Read the model definition and answer for the solid it produces. Units are mm, in the model's axes. A direction names the side the tool comes from. Coordinates: 2 decimals unless noted, no trailing zeros. Loops run counter-clockwise (first coordinate to the right, second up) from the corner with the lowest first, then second, coordinate; pieces in that order, holes last. Notation, with made-up numbers: M -19,45 L 4,45 A32 cw 4,80 Z; hole C -17.5,-34.5 d8. An arc over 180 degrees is marked long. One line per item, written item: value. Start each with the question number.
```python
from build123d import *

# Parameters (mm, degrees)
EXTRUDE_1_DEPTH     = 3
FILLET_1_R          = 5
SKETCH_4_R          = 1.75
SKETCH_4_R_2        = 1.35
CUT_EXTRUDE_2_DEPTH = 10
CUT_EXTRUDE_3_DEPTH = 10
SKETCH_5_R          = 1.6
CUT_EXTRUDE_4_DEPTH = 10


with BuildPart() as part:
    # Sketch 1 → Extrude 1 (new body)
    with BuildSketch(Plane(origin=(0, 0, 0), x_dir=(1, 0, 0), z_dir=(0, 1, 0))):
        Polygon((-84.734156599, 82.359506041), (109.265843401, 82.359506041), (109.265843401, 107.359506041), (137.265843401, 107.359506041), (137.265843401, 82.359506041), (137.265843401, -67.640493959), (-112.734156599, -67.640493959), (-112.734156599, 55.552013884), (-112.734156599, 107.359506041), (-84.734156599, 107.359506041), align=None)
    extrude(amount=EXTRUDE_1_DEPTH)

    # Fillet 1
    fillet_1_edges = [part.edges().sort_by_distance(p)[0] for p in [
        (137.265843401, 1.5, 67.640493959),
        (-112.734156599, 1.5, 67.640493959),
        (-112.734156599, 1.5, -107.359506041),
        (-84.734156599, 1.5, -107.359506041),
        (-84.734156599, 1.5, -82.359506041),
        (109.265843401, 1.5, -82.359506041),
        (109.265843401, 1.5, -107.359506041),
        (137.265843401, 1.5, -107.359506041),
    ]]
    fillet(fillet_1_edges, radius=FILLET_1_R)

    # Sketch 4 → Cut-Extrude 2 (cut)
    with BuildSketch(Plane(origin=(0, 3, 0), x_dir=(1, 0, 0), z_dir=(0, 1, 0))):
        with Locations(Location((12.608682616, 49.5, 0), (0, 0, 270))):
            Circle(SKETCH_4_R)
        with Locations(Location((-18.891317384, -14.5, 0), (0, 0, 270))):
            Circle(SKETCH_4_R)
        with Locations(Location((-42.582797937, 49.995, 0), (0, 0, 270))):
            Circle(SKETCH_4_R_2)
        with Locations(Location((-78.582797937, 13.995, 0), (0, 0, 270))):
            Circle(SKETCH_4_R_2)
        with Locations(Location((-42.582797937, 13.995, 0), (0, 0, 270))):
            Circle(SKETCH_4_R_2)
        with Locations(Location((12.608682616, -14.5, 0), (0, 0, 270))):
            Circle(SKETCH_4_R)
        with Locations(Location((-18.891317384, 49.5, 0), (0, 0, 270))):
            Circle(SKETCH_4_R)
        with Locations(Location((-78.582797937, 49.995, 0), (0, 0, 270))):
            Circle(SKETCH_4_R_2)
    extrude(amount=-CUT_EXTRUDE_2_DEPTH, mode=Mode.SUBTRACT)

    # Sketch 4_3 → Cut-Extrude 3 (cut)
    with BuildSketch(Plane(origin=(0, 3, 0), x_dir=(1, 0, 0), z_dir=(0, 1, 0))):
        with BuildLine():
            Line((57.265843401, 74.859506041), (107.265843401, 74.859506041))
            ThreePointArc((107.265843401, 74.859506041), (109.765843401, 72.359506041), (107.265843401, 69.859506041))
            Line((107.265843401, 69.859506041), (57.265843401, 69.859506041))
            ThreePointArc((57.265843401, 69.859506041), (54.765843401, 72.359506041), (57.265843401, 74.859506041))
        make_face()
        with BuildLine():
            Line((57.265843401, 59.859506041), (107.265843401, 59.859506041))
            ThreePointArc((107.265843401, 59.859506041), (109.765843401, 57.359506041), (107.265843401, 54.859506041))
            Line((107.265843401, 54.859506041), (57.265843401, 54.859506041))
            ThreePointArc((57.265843401, 54.859506041), (54.765843401, 57.359506041), (57.265843401, 59.859506041))
        make_face()
        with BuildLine():
            Line((57.265843401, 44.859506041), (107.265843401, 44.859506041))
            ThreePointArc((107.265843401, 44.859506041), (109.765843401, 42.359506041), (107.265843401, 39.859506041))
            Line((107.265843401, 39.859506041), (57.265843401, 39.859506041))
            ThreePointArc((57.265843401, 39.859506041), (54.765843401, 42.359506041), (57.265843401, 44.859506041))
        make_face()
        with BuildLine():
            Line((57.265843401, 29.859506041), (107.265843401, 29.859506041))
            ThreePointArc((107.265843401, 29.859506041), (109.765843401, 27.359506041), (107.265843401, 24.859506041))
            Line((107.265843401, 24.859506041), (57.265843401, 24.859506041))
            ThreePointArc((57.265843401, 24.859506041), (54.765843401, 27.359506041), (57.265843401, 29.859506041))
        make_face()
        with BuildLine():
            Line((57.265843401, 14.859506041), (107.265843401, 14.859506041))
            ThreePointArc((107.265843401, 14.859506041), (109.765843401, 12.359506041), (107.265843401, 9.859506041))
            Line((107.265843401, 9.859506041), (57.265843401, 9.859506041))
            ThreePointArc((57.265843401, 9.859506041), (54.765843401, 12.359506041), (57.265843401, 14.859506041))
        make_face()
        with BuildLine():
            Line((57.265843401, -0.140493959), (107.265843401, -0.140493959))
            ThreePointArc((107.265843401, -0.140493959), (109.765843401, -2.640493959), (107.265843401, -5.140493959))
            Line((107.265843401, -5.140493959), (57.265843401, -5.140493959))
            ThreePointArc((57.265843401, -5.140493959), (54.765843401, -2.640493959), (57.265843401, -0.140493959))
        make_face()
        with BuildLine():
            Line((57.265843401, -15.140493959), (107.265843401, -15.140493959))
            ThreePointArc((107.265843401, -15.140493959), (109.765843401, -17.640493959), (107.265843401, -20.140493959))
            Line((107.265843401, -20.140493959), (57.265843401, -20.140493959))
            ThreePointArc((57.265843401, -20.140493959), (54.765843401, -17.640493959), (57.265843401, -15.140493959))
        make_face()
        with BuildLine():
            Line((57.265843401, -30.140493959), (107.265843401, -30.140493959))
            ThreePointArc((107.265843401, -30.140493959), (109.765843401, -32.640493959), (107.265843401, -35.140493959))
            Line((107.265843401, -35.140493959), (57.265843401, -35.140493959))
            ThreePointArc((57.265843401, -35.140493959), (54.765843401, -32.640493959), (57.265843401, -30.140493959))
        make_face()
        with BuildLine():
            Line((57.265843401, -45.140493959), (107.265843401, -45.140493959))
            ThreePointArc((107.265843401, -45.140493959), (109.765843401, -47.640493959), (107.265843401, -50.140493959))
            Line((107.265843401, -50.140493959), (57.265843401, -50.140493959))
            ThreePointArc((57.265843401, -50.140493959), (54.765843401, -47.640493959), (57.265843401, -45.140493959))
        make_face()
        with BuildLine():
            Line((-12.734156599, 74.859506041), (37.265843401, 74.859506041))
            ThreePointArc((37.265843401, 74.859506041), (39.765843401, 72.359506041), (37.265843401, 69.859506041))
            Line((37.265843401, 69.859506041), (-12.734156599, 69.859506041))
            ThreePointArc((-12.734156599, 69.859506041), (-15.234156599, 72.359506041), (-12.734156599, 74.859506041))
        make_face()
        with BuildLine():
            Line((-12.734156599, 59.859506041), (37.265843401, 59.859506041))
            ThreePointArc((37.265843401, 59.859506041), (39.765843401, 57.359506041), (37.265843401, 54.859506041))
            Line((37.265843401, 54.859506041), (-12.734156599, 54.859506041))
            ThreePointArc((-12.734156599, 54.859506041), (-15.234156599, 57.359506041), (-12.734156599, 59.859506041))
        make_face()
        with BuildLine():
            Line((-82.734156599, 59.859506041), (-32.734156599, 59.859506041))
            ThreePointArc((-32.734156599, 59.859506041), (-30.234156599, 57.359506041), (-32.734156599, 54.859506041))
            Line((-32.734156599, 54.859506041), (-82.734156599, 54.859506041))
            ThreePointArc((-82.734156599, 54.859506041), (-85.234156599, 57.359506041), (-82.734156599, 59.859506041))
        make_face()
        with BuildLine():
            Line((-12.734156599, -45.140493959), (37.265843401, -45.140493959))
            ThreePointArc((37.265843401, -45.140493959), (39.765843401, -47.640493959), (37.265843401, -50.140493959))
            Line((37.265843401, -50.140493959), (-12.734156599, -50.140493959))
            ThreePointArc((-12.734156599, -50.140493959), (-15.234156599, -47.640493959), (-12.734156599, -45.140493959))
        make_face()
        with BuildLine():
            Line((-82.734156599, -45.140493959), (-32.734156599, -45.140493959))
            ThreePointArc((-32.734156599, -45.140493959), (-30.234156599, -47.640493959), (-32.734156599, -50.140493959))
            Line((-32.734156599, -50.140493959), (-82.734156599, -50.140493959))
            ThreePointArc((-82.734156599, -50.140493959), (-85.234156599, -47.640493959), (-82.734156599, -45.140493959))
        make_face()
        with BuildLine():
            Line((-82.734156599, -30.140493959), (-32.734156599, -30.140493959))
            ThreePointArc((-32.734156599, -30.140493959), (-30.234156599, -32.640493959), (-32.734156599, -35.140493959))
            Line((-32.734156599, -35.140493959), (-82.734156599, -35.140493959))
            ThreePointArc((-82.734156599, -35.140493959), (-85.234156599, -32.640493959), (-82.734156599, -30.140493959))
        make_face()
        with BuildLine():
            Line((-82.734156599, -15.140493959), (-32.734156599, -15.140493959))
            ThreePointArc((-32.734156599, -15.140493959), (-30.234156599, -17.640493959), (-32.734156599, -20.140493959))
            Line((-32.734156599, -20.140493959), (-82.734156599, -20.140493959))
            ThreePointArc((-82.734156599, -20.140493959), (-85.234156599, -17.640493959), (-82.734156599, -15.140493959))
        make_face()
    extrude(amount=-CUT_EXTRUDE_3_DEPTH, mode=Mode.SUBTRACT)

    # Sketch 5 → Cut-Extrude 4 (cut)
    with BuildSketch(Plane(origin=(0, 3, 0), x_dir=(1, 0, 0), z_dir=(0, 1, 0))):
        with Locations(Location((-97.734156599, 67.359506041, 0), (0, 0, 270))):
            Circle(SKETCH_5_R)
        with Locations(Location((-97.734156599, 27.359506041, 0), (0, 0, 270))):
            Circle(SKETCH_5_R)
        with Locations(Location((-97.734156599, -12.640493959, 0), (0, 0, 270))):
            Circle(SKETCH_5_R)
        with Locations(Location((-97.734156599, -52.640493959, 0), (0, 0, 270))):
            Circle(SKETCH_5_R)
        with Locations(Location((122.265843401, -52.640493959, 0), (0, 0, 270))):
            Circle(SKETCH_5_R)
        with Locations(Location((122.265843401, -12.640493959, 0), (0, 0, 270))):
            Circle(SKETCH_5_R)
        with Locations(Location((122.265843401, 27.359506041, 0), (0, 0, 270))):
            Circle(SKETCH_5_R)
        with Locations(Location((122.265843401, 67.359506041, 0), (0, 0, 270))):
            Circle(SKETCH_5_R)
    extrude(amount=-CUT_EXTRUDE_4_DEPTH, mode=Mode.SUBTRACT)


solid = part.part
```
1) Consider line 1 along Z through (x, y) = (7, 2.7); line 2 along Z through (x, y) = (-37, 1.15); line 3 along Z through (x, y) = (-97.5, 0.7). Determine where each line is inside the solid, lowest interval first.
2) A tool of negligible diameter and unlimited length cuts with its end or side. For faces 1 (the face through (14, 3, -21)), 2 (the face through (110.692, 1.521, -105.856)), from which of +Z, -Z, +X, -X, +Y, -Y can it reach the whole face along a straight path? Write none if from no direction.
3) Section D-D (x = 71) is taken. Count the separate pieces of the cut face and the enclosed holes in it, then the cut area to 3 significant figures.
4) For a pull along X with two mould halves and no side action, classify faces 3 (the face through (-86.238, 1.521, -105.934)), 4 (the face through (14, 0, -21)), 5 (the face through (135.762, 1.521, -105.934)) as released by +X, released by -X, zero draft, split by the parting line, or undercut.
5) Section B-B (x = 32) is taken. Determine the outline of the cut face in (y, z).
6) Section A-A (z = -92.5) is taken. Determine the outline of the cut face in (x, y).
7) Flat-ended cylindrical pins translate along their axes: pin 1 (2.5 mm diameter, centred on x = 122.27, z = -67.36, fed in from -Y); pin 2 (0.9 mm diameter, centred on x = -47.5, y = 2, fed in from -Z). Find the tip coordinate at first contact, or state that the pin passes through.
8) Section C-C (x = -56) is taken. Determine the outline of the cut face in (y, z), then the cut area to 3 significant figures.
Results found:
1. line 1: z = -82.36 to -74.86, -69.86 to -59.86, -54.86 to 45.14, 50.14 to 67.64
1. line 2: z = -82.36 to -59.86, -54.86 to 15.14, 20.14 to 30.14, 35.14 to 45.14, 50.14 to 67.64
1. line 3: z = -107.36 to -68.94, -65.78 to -28.94, -25.78 to 11.06, 14.22 to 51.06, 54.22 to 67.64
2. face 1: +Z, -Z, +X, -X, +Y
2. face 2: -Z, +Y, -Y
3. separate pieces: 10
3. enclosed holes: 0
3. area: 315 mm²
4. face 3: undercut
4. face 4: zero draft
4. face 5: released by +X
5. outline: M 0,-82.36 L 3,-82.36 L 3,-74.86 L 0,-74.86 Z; M 0,-69.86 L 3,-69.86 L 3,-59.86 L 0,-59.86 Z; M 0,-54.86 L 3,-54.86 L 3,45.14 L 0,45.14 Z; M 0,50.14 L 3,50.14 L 3,67.64 L 0,67.64 Z
6. outline: M -112.73,0 L -84.73,0 L -84.73,3 L -112.73,3 Z; M 109.27,0 L 137.27,0 L 137.27,3 L 109.27,3 Z
7. pin 1: passes through
7. pin 2: stops at z = -82.36
8. outline: M 0,-82.36 L 3,-82.36 L 3,-59.86 L 0,-59.86 Z; M 0,-54.86 L 3,-54.86 L 3,15.14 L 0,15.14 Z; M 0,20.14 L 3,20.14 L 3,30.14 L 0,30.14 Z; M 0,35.14 L 3,35.14 L 3,45.14 L 0,45.14 Z; M 0,50.14 L 3,50.14 L 3,67.64 L 0,67.64 Z
8. area: 390 mm²
